```python
from build123d import *

# Parameters (mm, degrees)
F0_R        = 5
F1_DEPTH    = 5
F2_R        = 1.25
F3_DEPTH    = 100
F4_S5_R     = 1.25
F4_T6_DEPTH = 9


# Not quite as in the source:
# - a fillet or chamfer that OpenCascade refuses, or shapes differently, is made with other operations: its cross-section is extruded or revolved along the edge and cut away or added


with BuildPart() as f1:
    # F0 (on Front) → F1 (new body)
    with BuildSketch(Plane.XZ):
        Circle(F0_R)
    extrude(amount=F1_DEPTH)

    # F2 (on face) → F3 (join)
    with BuildSketch(Plane.XZ.offset(5)):
        Circle(F2_R)
    extrude(amount=F3_DEPTH)

    # F4: chamfer of 4 on 1 edges, made by hand


with BuildPart() as f4_tool2:
    # F4_s3 → F4_t4 (revolve)
    with BuildSketch(Plane.XY):
        Polygon((5, -1), (1, -5), (5, -5), align=None)
    revolve(axis=Axis((0, -5, 0), (0, -1, 0)))

    # F4_s5 → F4_t6 (cut, symmetric)
    with BuildSketch(Plane.XZ.offset(3)):
        Circle(F4_S5_R)
    extrude(amount=F4_T6_DEPTH, both=True, mode=Mode.SUBTRACT)


with BuildPart() as f1_1:
    add(f1.part)

    # F4_t1: cut F4_tool2
    add(f4_tool2.part, mode=Mode.SUBTRACT)


solid = f1_1.part
```
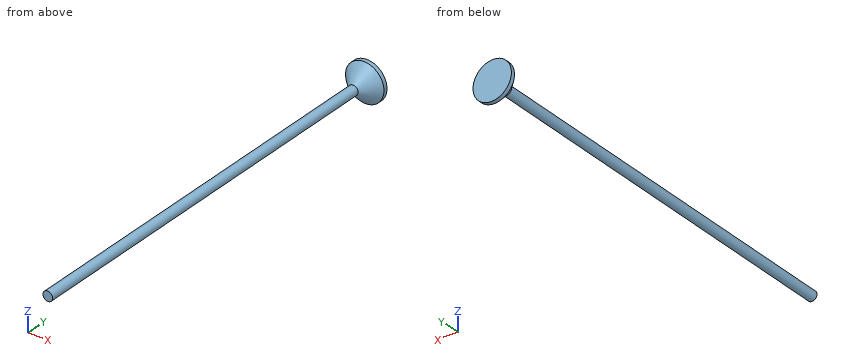
Can you work these out from the model? Positions are in its coordinate system, mm. Give positions to 0.01 mm unless a question says otherwise; leave off trailing zeros. Order: outer loops, then holes, each group sorted by start corner. A loop starts at its lowest first (then second) coordinate and runs counter-clockwise, first axis right, second up. Notation, with made-up numbers: M 23.5,-11.75 L 69.5,-11.75 A22 cw 69.5,16.25 Z; hole C -19.5,-1.75 d11. An arc over 180 degrees is marked long. One line per item, written item: value.
1) For P1, Ø1, axis at x = 3.5, z = -2, coming from the -Y side; P2, Ø5, axis at y = -65, z = -1.5, coming from the +X side; P3, Ø2, axis at x = 2.5, y = -14, coming from the +Z side; P4, Ø6, axis at x = 3, y = -21.5, coming from the +Z side, each with a flat end and sliding along its axis, tell me the tip position at first contact or that it passes through.
Answer sheet:
P1: stops at y = -2.47
P2: stops at x = 1.25
P3: passes through
P4: stops at z = 1.25
2) I want a section at A-A, the plane x = 0. List the corners of the cut face in (y, z) for me.
Answer sheet:
outline: M -105,-1.25 L -4.75,-1.25 L -1,-5 L 0,-5 L 0,5 L -1,5 L -4.75,1.25 L -105,1.25 Z
3) I want a section at C-C, the plane y = -25. List the corners of the cut face in (x, z) for me, plus the area to 3 significant figures.
Answer sheet:
outline: C 0,0 d2.5
area: 4.91 mm^2
4) Please list where these lines run through material, in increasing order: line 1 along X through (y, z) = (-42.5, 0.5); line 2 along X through (y, z) = (-39, 0.75); line 3 along Y through (x, z) = (2.5, 2.25).
Answer sheet:
line 1: x = -1.15 to 1.15
line 2: x = -1 to 1
line 3: y = -2.64 to 0
5) I want a section at B-B, the plane z = 0. List the corners of the cut face in (x, y) for me, plus the area to 3 significant figures.
Answer sheet:
outline: M -5,-1 L -1.25,-4.75 L -1.25,-105 L 1.25,-105 L 1.25,-4.75 L 5,-1 L 5,0 L -5,0 Z
area: 284 mm^2
